```python
from build123d import *

# Parameters (mm, degrees)
SKETCH1_R                 = 2.65
F_30_X_60G_X_R1_5_1_DEPTH = 220


with BuildPart() as part:
    # Sketch1 → 铝型材 30 X 60G X R1.5(1) (new body)
    with BuildSketch(Plane(origin=(0, 0, 0), x_dir=(0, 0, -1), z_dir=(1, 0, 0))):
        with BuildLine():
            Line((-3.25, 30), (-3.25, 29))
            Line((-3.25, 29), (-4.25, 29))
            Line((-4.25, 29), (-4.25, 21.277812156))
            ThreePointArc((-4.25, 21.277812156), (0, 20.5), (4.25, 21.277812156))
            Line((4.25, 21.277812156), (4.25, 29))
            Line((4.25, 29), (3.25, 29))
            Line((3.25, 29), (3.25, 30))
            Line((3.25, 30), (13.5, 30))
            ThreePointArc((13.5, 30), (14.560660172, 29.560660172), (15, 28.5))
            Line((15, 28.5), (15, 18.25))
            Line((15, 18.25), (14, 18.25))
            Line((14, 18.25), (14, 19.25))
            Line((14, 19.25), (6.277812156, 19.25))
            ThreePointArc((6.277812156, 19.25), (5.5, 15), (6.277812156, 10.75))
            Line((6.277812156, 10.75), (14, 10.75))
            Line((14, 10.75), (14, 11.75))
            Line((14, 11.75), (15, 11.75))
            Line((15, 11.75), (15, -11.75))
            Line((15, -11.75), (14, -11.75))
            Line((14, -11.75), (14, -10.75))
            Line((14, -10.75), (6.277812156, -10.75))
            ThreePointArc((6.277812156, -10.75), (5.5, -15), (6.277812156, -19.25))
            Line((6.277812156, -19.25), (14, -19.25))
            Line((14, -19.25), (14, -18.25))
            Line((14, -18.25), (15, -18.25))
            Line((15, -18.25), (15, -28.5))
            ThreePointArc((15, -28.5), (14.560660172, -29.560660172), (13.5, -30))
            Line((13.5, -30), (3.25, -30))
            Line((3.25, -30), (3.25, -29))
            Line((3.25, -29), (4.25, -29))
            Line((4.25, -29), (4.25, -21.277812156))
            ThreePointArc((4.25, -21.277812156), (0, -20.5), (-4.25, -21.277812156))
            Line((-4.25, -21.277812156), (-4.25, -29))
            Line((-4.25, -29), (-3.25, -29))
            Line((-3.25, -29), (-3.25, -30))
            Line((-3.25, -30), (-13.5, -30))
            ThreePointArc((-13.5, -30), (-14.560660172, -29.560660172), (-15, -28.5))
            Line((-15, -28.5), (-15, -18.25))
            Line((-15, -18.25), (-14, -18.25))
            Line((-14, -18.25), (-14, -19.25))
            Line((-14, -19.25), (-6.277812156, -19.25))
            ThreePointArc((-6.277812156, -19.25), (-5.5, -15), (-6.277812156, -10.75))
            Line((-6.277812156, -10.75), (-14, -10.75))
            Line((-14, -10.75), (-14, -11.75))
            Line((-14, -11.75), (-15, -11.75))
            Line((-15, -11.75), (-15, 11.75))
            Line((-15, 11.75), (-14, 11.75))
            Line((-14, 11.75), (-14, 10.75))
            Line((-14, 10.75), (-6.277812156, 10.75))
            ThreePointArc((-6.277812156, 10.75), (-5.5, 15), (-6.277812156, 19.25))
            Line((-6.277812156, 19.25), (-14, 19.25))
            Line((-14, 19.25), (-14, 18.25))
            Line((-14, 18.25), (-15, 18.25))
            Line((-15, 18.25), (-15, 28.5))
            ThreePointArc((-15, 28.5), (-14.560660172, 29.560660172), (-13.5, 30))
            Line((-13.5, 30), (-3.25, 30))
        make_face()
        with Locations((-11, 26)):
            Circle(SKETCH1_R, mode=Mode.SUBTRACT)
        with Locations((11, 26)):
            Circle(SKETCH1_R, mode=Mode.SUBTRACT)
        with Locations((11, -26)):
            Circle(SKETCH1_R, mode=Mode.SUBTRACT)
        with Locations((-11, -26)):
            Circle(SKETCH1_R, mode=Mode.SUBTRACT)
        with BuildLine():
            Line((-12.5, 7.5), (-4, 7.5))
            Line((-4, 7.5), (-1.665625283, 13.135679101))
            ThreePointArc((-1.665625283, 13.135679101), (0, 17.5), (1.665625283, 13.135679101))
            Line((1.665625283, 13.135679101), (4, 7.5))
            Line((4, 7.5), (12.5, 7.5))
            Line((12.5, 7.5), (12.5, -7.5))
            Line((12.5, -7.5), (4, -7.5))
            Line((4, -7.5), (1.665625283, -13.135679101))
            ThreePointArc((1.665625283, -13.135679101), (0, -17.5), (-1.665625283, -13.135679101))
            Line((-1.665625283, -13.135679101), (-4, -7.5))
            Line((-4, -7.5), (-12.5, -7.5))
            Line((-12.5, -7.5), (-12.5, 7.5))
        make_face(mode=Mode.SUBTRACT)
    extrude(amount=F_30_X_60G_X_R1_5_1_DEPTH)


solid = part.part
```
Check sheet for the modelled part. Datum: model origin and axes. Units: mm. A direction names the side the tool comes from. Coordinates: 2 decimals unless noted, no trailing zeros. Loops run counter-clockwise (first coordinate to the right, second up) from the corner with the lowest first, then second, coordinate; pieces in that order, holes last.
1) Sectioned sample at A-A (y = 26). Record the boundary of the cut face in (x, z).
2) Access from +Z, -Z, +X, -X, +Y, -Y to the whole of each face (thin tool, end or side, straight path). Record for faces 5 (the face through (108, 23, -15)), 6 (the face through (108.5, -14.9, -5.5)).
3) Gauge pin test, flat ends, axial feed: pin 1 (0.5 mm diameter, centred on x = 151, y = 29.5, fed in from -Z); pin 2 (1.1 mm diameter, centred on x = 64.5, z = 14.5, fed in from +Y); pin 3 (0.8 mm diameter, centred on x = 161, z = -14.5, fed in from -Y). Record the tip position at first contact, or that the pin passes through.
4) Sectioned sample at D-D (y = -5). Record the boundary of the cut face in (x, z).
5) Material ranges on probe 1 along Y at (x, z) = (26, 10.75); probe 2 along Y at (x, z) = (19.5, -10.25); probe 3 along Z at (x, y) = (38, 23), recorded low to high.
6) Release check for a two-part mould opening along Y. For faces 1 (the face through (108.46, 23.41, -10.43)), 2 (the face through (108, 23, 15)), 3 (the face through (108, 30, -8)), 4 (the face through (108.5, -10.4, 2.8)) record: released by +Y, released by -Y, zero draft, split by the parting line, or undercut.
7) Sectioned sample at B-B (y = 15). Record the boundary of the cut face in (x, z).
8) Sectioned sample at C-C (x = 57). Count the separate pieces of the cut face and the enclosed holes in it, and give its area (3 significant figures).
Check sheet entries:
1. outline: (0, -15) - (220, -15) - (220, -13.65) - (0, -13.65) - close; (0, -8.35) - (220, -8.35) - (220, -4.25) - (0, -4.25) - close; (0, 4.25) - (220, 4.25) - (220, 8.35) - (0, 8.35) - close; (0, 13.65) - (220, 13.65) - (220, 15) - (0, 15) - close
2. face 5: -Z, +X, -X, +Y, -Y
2. face 6: +X, -X
3. pin 1: stops at z = -14.8
3. pin 2: stops at y = 29.93
3. pin 3: stops at y = -29.87
4. outline: (0, -15) - (220, -15) - (220, -12.5) - (0, -12.5) - close; (0, 12.5) - (220, 12.5) - (220, 15) - (0, 15) - close
5. probe 1: y = -30 to -28.64, -23.36 to -19.25, -10.75 to -7.5, 7.5 to 10.75, 19.25 to 23.36, 28.64 to 30
5. probe 2: y = -30 to -28.54, -23.46 to -19.25, -10.75 to -7.5, 7.5 to 10.75, 19.25 to 23.46, 28.54 to 30
5. probe 3: z = -15 to -4.25, 4.25 to 15
6. face 1: undercut
6. face 2: zero draft
6. face 3: released by +Y
6. face 4: undercut
7. outline: (0, -5.5) - (220, -5.5) - (220, -2.5) - (0, -2.5) - close; (0, 2.5) - (220, 2.5) - (220, 5.5) - (0, 5.5) - close
8. separate pieces: 1
8. enclosed holes: 5
8. area: 775 mm2
